```python
from build123d import *
from OCP.BRepFilletAPI import BRepFilletAPI_MakeChamfer

# Parameters (mm, degrees)
CUT_EXTRUDE1_DEPTH = 28.123421613
SKETCH3_R          = 2
CUT_EXTRUDE2_DEPTH = 2
CHAMFER1_SIZE      = 0.8
CHAMFER1_SIZE2     = 0.984433479
CHAMFER1_SIZE2_2   = 0.691197975


with BuildPart() as part:
    # Sketch1 → Revolve1 (revolve)
    with BuildSketch(Plane.XY, mode=Mode.PRIVATE) as revolve1_sk:
        Polygon((0, 0), (-17.2, 0), (-15.1, -12), (0, -12), align=None)
    revolve(revolve1_sk.sketch.rotate(Axis((0, 0, 0), (0, -1, 0)), 270), axis=Axis((0, 0, 0), (0, -1, 0)))

    # Sketch2 → Cut-Extrude1 (cut, through all)
    with BuildSketch(Plane(origin=(0, 0, 0), x_dir=(1, 0, 0), z_dir=(0, 1, 0))):
        with BuildLine():
            Line((-9.1, -5.8), (-7.3, -5.8))
            Line((-7.3, -5.8), (-7.3, -10.756858277))
            ThreePointArc((-7.3, -10.756858277), (0, -13), (7.3, -10.756858277))
            Line((7.3, -10.756858277), (7.3, -5.8))
            Line((7.3, -5.8), (9.1, -5.8))
            Line((9.1, -5.8), (9.1, -4))
            Line((9.1, -4), (7.3, -4))
            Line((7.3, -4), (7.3, 0))
            Line((7.3, 0), (13, 0))
            ThreePointArc((13, 0), (0, 13), (-13, 0))
            Line((-13, 0), (-7.3, 0))
            Line((-7.3, 0), (-7.3, -4))
            Line((-7.3, -4), (-9.1, -4))
            Line((-9.1, -4), (-9.1, -5.8))
        make_face()
    extrude(amount=-CUT_EXTRUDE1_DEPTH, mode=Mode.SUBTRACT)

    # Sketch3 → Cut-Extrude2 (cut)
    with BuildSketch(Plane(origin=(0, 0, 0), x_dir=(1, 0, 0), z_dir=(0, 1, 0))):
        with Locations((-8.1, -4.9)):
            Circle(SKETCH3_R)
        with Locations((8.1, -4.9)):
            Circle(SKETCH3_R)
    extrude(amount=-CUT_EXTRUDE2_DEPTH, mode=Mode.SUBTRACT)

    # Chamfer1: one chamfer whose edges measure the first distance from different faces: ONE call of the kernel's chamfer builder (chamfer() names one face for all edges)
    chamfer1_edges_1 = [part.edges().sort_by_distance(p)[0] for p in [
        (0, -12, -15.1),
    ]]
    chamfer1_side_1 = [part.faces().sort_by_distance(p)[0] for p in [
        (0, -12, -14.672907504),
    ]]
    chamfer1_edges_2 = [part.edges().sort_by_distance(p)[0] for p in [
        (0, 0, -17.2),
    ]]
    chamfer1_side_2 = [part.faces().sort_by_distance(p)[0] for p in [
        (0, -6, -16.15),
    ]]
    chamfer1 = BRepFilletAPI_MakeChamfer(part.part.solid().wrapped)
    for e in chamfer1_edges_1:
        chamfer1.Add(CHAMFER1_SIZE, CHAMFER1_SIZE2, e.wrapped, chamfer1_side_1[0].wrapped)  # the first distance lies on this face
    for e in chamfer1_edges_2:
        chamfer1.Add(CHAMFER1_SIZE, CHAMFER1_SIZE2_2, e.wrapped, chamfer1_side_2[0].wrapped)  # the first distance lies on this face
    add(Compound.cast(chamfer1.Shape()), mode=Mode.REPLACE)


solid = part.part
```
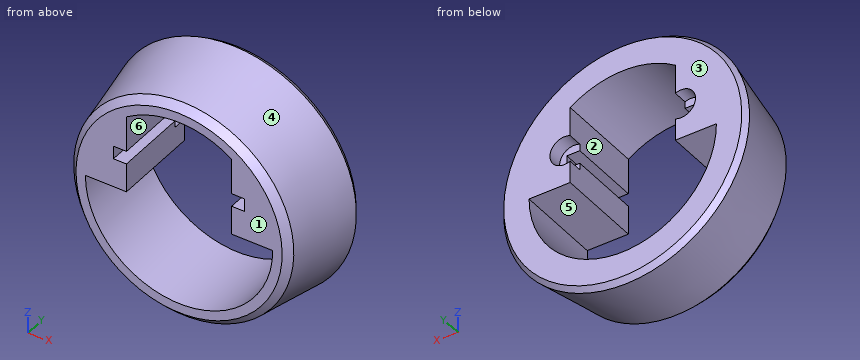
The model under review builds one solid part; all positions refer to its coordinate system, in mm. Face numbers are marked on the shaded views. A direction names the side the tool comes from. Give positions to 0.01 mm unless a question says otherwise; leave off trailing zeros. Loops run counter-clockwise (first coordinate to the right, second up) from the corner with the lowest first, then second, coordinate; pieces in that order, holes last. Notation, with made-up numbers: (36.25, 70) - (83.25, 70) arc R16 cw to (83.25, 76) - close; hole circle Ø8 at (83.5, -37). An arc over 180 degrees is marked (long way). Answer as a JSON object with one key per item and string values.
Q1. Add section A-A on x = 0. State the section outline as (y, z) points, plus the area to 3 significant figures.
Worked out:
{"outline": "(-12, -14.3) - (-11.03, -15.27) - (-0.79, -17.06) - (0, -16.51) - (0, -13) - (-12, -13) - close; (-12, 13) - (0, 13) - (0, 16.51) - (-0.79, 17.06) - (-11.03, 15.27) - (-12, 14.3) - close", "area": "74.3 mm^2"}
Q2. Add section D-D on x = 8.1. Count the separate pieces of the cut face and the enclosed holes in it, plus the area to 3 significant figures.
Worked out:
{"separate pieces": "3", "enclosed holes": "0", "area": "186 mm^2"}
Q3. Add section B-B on y = -9.5. State the section outline as (x, z) points (1 decimal), plus the area to 3 significant figures.
Worked out:
{"outline": "circle Ø31.1 at (0, 0); hole (-13, 0) arc R13 ccw to (13, 0) - (7.3, 0) - (7.3, 4) - (9.1, 4) - (9.1, 5.8) - (7.3, 5.8) - (7.3, 10.8) arc R13 ccw to (-7.3, 10.8) - (-7.3, 5.8) - (-9.1, 5.8) - (-9.1, 4) - (-7.3, 4) - (-7.3, 0) - close", "area": "307 mm^2"}
Q4. For the marked faces 1 and 2, list the 3-axis set-ups (+Z, -Z, +X, -X, +Y, -Y) from which the entire face can be reached by the end or side of a thin tool; tool diameter is ignored.
Worked out:
{"face 1": "+Z, -Z, +X, -X, -Y", "face 2": "+Y, -Y"}
Q5. To check wall thickness, follow line 1 along Z through (x, y) = (8.1, -0.6); line 2 along Z through (x, y) = (-8.1, -0.95); line 3 along X through (y, z) = (-3.5, -3). State the ranges of each line that lie inside material, in increasing order.
Worked out:
{"line 1": "z = -14.87 to -10.17, 0 to 2.9, 6.9 to 14.87", "line 2": "z = -14.98 to -10.17, 0 to 2.9, 6.9 to 14.98", "line 3": "x = -16.31 to -12.65, 12.65 to 16.31"}
Q6. Add section C-C on y = -1.5. State the section outline as (x, z) points (1 decimal), plus the area to 3 significant figures.
Worked out:
{"outline": "circle Ø33.9 at (0, 0); hole (-13, 0) arc R13 ccw to (13, 0) - (7.3, 0) - (7.3, 3.1) arc R2 ccw (long way) to (7.3, 6.7) - (7.3, 10.8) arc R13 ccw to (-7.3, 10.8) - (-7.3, 6.7) arc R2 ccw (long way) to (-7.3, 3.1) - (-7.3, 0) - close", "area": "438 mm^2"}
Q7. Mouldability with a two-part tool opening along Z and no side actions: class the marked faces 3, 4, 5 and 6 as +Z half, -Z half, draft (parallel to the pull), parting line (faces both ways), or undercut.
Worked out:
{"face 3": "draft", "face 4": "parting line", "face 5": "undercut", "face 6": "undercut"}
Q8. Insertion check: pin 1 (2.5 mm diameter, centred on x = -8.1, z = 4.9, fed in from +Y); pin 2 (1.4 mm diameter, centred on y = -9, z = 5, fed in from -X); pin 3 (4 mm diameter, centred on x = -4.5, z = 7, fed in from -Y); pin 4 (5 mm diameter, centred on x = -6.5, y = -8.5, fed in from -Z). Each pin has a flat end and moves straight along its axis. Give the tip position at first contact, or say it passes through.
Worked out:
{"pin 1": "stops at y = -2", "pin 2": "stops at x = -15.06", "pin 3": "passes through", "pin 4": "stops at z = -15.33"}
